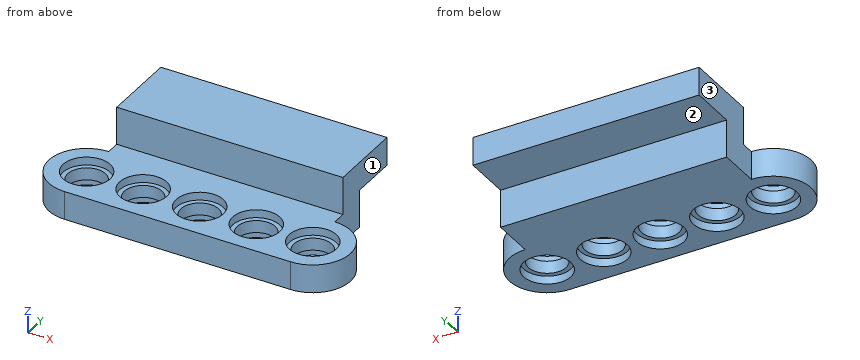
Autodesk Inventor part; units mm, degrees
ref_plane "YZ Plane" through (0, 0, 0) normal (1, 0, 0) x (0, 1, 0)
ref_plane "XZ Plane" through (0, 0, 0) normal (0, 1, 0) x (-1, 0, 0)
ref_plane "XY Plane" through (0, 0, 0) normal (0, 0, 1) x (1, 0, 0)
sketch "Sketch1" plane through (0, 0, 0) normal (0, 0, 1) x (1, 0, 0)
  arc A0 (-15, 4) -> (-15, -4) centre (-15, 0) ccw
  line L0 (-5, -4) -> (-15, -4)
  line L1 (-3, 0) -> (-3, 5.2247) construction
  arc A1 (9, -4) -> (9, 4) centre (9, 0) ccw
  line L2 (-5, -4) -> (9, -4)
  line L3 (9, 8.4612) -> (-15, 8.4612)
  line L4 (-15, 8.4612) -> (-15, 4)
  line L5 (9, 4) -> (9, 8.4612)
  dimension "d11" = 4
extrude "Extrusion1" add sketch "Sketch1" along normal blind 3
sketch "Sketch2" plane through (0, 0, 3) normal (0, 0, 1) x (1, 0, 0)
  arc A0 (-15, 4) -> (-15, -4) centre (-15, 0) ccw
  point P0 (0, 0)
hole "Hole1" at (-15, 0, 3) direction (0, 0, -1) diameter 4 depth 3 tip angle 118 counterbore diameter 5 counterbore depth 0.85
sketch "Sketch5" plane through (0, 0, 0) normal (0, 0, -1) x (-1, 0, 0)
  circle A0 centre (15, 0) radius 2
  circle A1 centre (15, 0) radius 2.5
  point P0 (0, 0)
extrude "Extrusion3" cut sketch "Sketch5" against normal blind 0.85
pattern_linear "Rectangular Pattern2" count 5 spacing 6 along (1, 0, 0) of "Extrusion3", "Hole1"
sketch "Sketch6" plane through (0, 0, 3) normal (0, 0, 1) x (1, 0, 0)
  point P0 (0, 0)
sketch "Sketch7" plane through (0, 0, 3) normal (0, 0, 1) x (1, 0, 0)
  line L0 (9, 4) -> (9, 8.4612)
  line L1 (-15, 8.4612) -> (9, 8.4612)
  line L2 (9, 8.4612) -> (9, 5.4612)
  line L3 (9, 5.4612) -> (-15, 5.4612)
  line L4 (-15, 5.4612) -> (-15, 8.4612)
  point P0 (0, 0)
  dimension "d24" = 3
extrude "Extrusion4" add sketch "Sketch7" along normal blind 4
sketch "Sketch8" plane through (-15, 8.4612, 0) normal (0, 1, 0) x (1, 0, 0)
  line L0 (24, -3) -> (24, -7)
  line L1 (0, -7) -> (24, -7)
  line L2 (24, -7) -> (24, -4)
  line L3 (24, -4) -> (0, -4)
  line L4 (0, -4) -> (0, -7)
  point P0 (15, 0)
  dimension "d27" = 3
extrude "Extrusion5" add sketch "Sketch8" along normal blind 5
properties part number "caster_pad"
Input: part model. Units: mm. Frame: model coordinates. Face numbers are marked on the shaded views. A direction names the side the tool comes from. Coordinates: 2 decimals unless noted, no trailing zeros. Loops run counter-clockwise (first coordinate to the right, second up) from the corner with the lowest first, then second, coordinate; pieces in that order, holes last. Notation, with made-up numbers: (47, -16) - (86, -16) arc R35 cw to (86, 22) - close; hole circle Ø8 at (69, -25.5). An arc over 180 degrees is marked (long way). Answer in a Markdown table with one row per item. Add a question column.
Item 1: Access query for the marked faces 1, 2 and 3. Directions: +Z, -Z, +X, -X, +Y, -Y. A direction counts if a zero-diameter tool reaches every point of the face in a straight line with its end or side. Return the directions, or none.
Item 2: Section query D-D on z = 5.75. Return the cut outline in (x, y), then the cut area to 3 significant figures.
Item 3: Contact query for flat-ended pins moving along their axis: P1, Ø1, axis at x = -14, y = -1.5, coming from the -Z side; P2, Ø2, axis at y = 6.5, z = 6, coming from the +X side; P3, Ø3, axis at y = 10, z = 5.5, coming from the -X side. Output: stop coordinate, or through.
Item 4: Section query B-B on y = 0. State how many separate pieces and enclosed holes the cut face has, then the cut area to 3 significant figures.
Item 5: Line query: line 1 along X through (y, z) = (0, 1.35); line 2 along X through (y, z) = (0, 2.6); line 3 along Y through (x, z) = (3, 0.25). Output: solid intervals per line, ascending. Write a range as [from, to].
Item 6: Section query C-C on y = 10. Return the cut outline in (x, z), then the cut area to 3 significant figures.
Item 7: Section query A-A on x = -6. Return the cut outline in (y, z).
Recorded:
| question | item | result |
|---|---|---|
| 1 | face 1 | +Z, -Z, +X, +Y |
| 1 | face 2 | -Z, +X, -X, +Y |
| 1 | face 3 | +Z, -Z, -X, +Y |
| 2 | outline | (-15, 5.46) - (9, 5.46) - (9, 13.46) - (-15, 13.46) - close |
| 2 | area | 192 mm^2 |
| 3 | P1 | z = 0.85 |
| 3 | P2 | x = 9 |
| 3 | P3 | x = -15 |
| 4 | separate pieces | 6 |
| 4 | enclosed holes | 0 |
| 4 | area | 27.5 mm^2 |
| 5 | line 1 | [-19, -17], [-13, -11], [-7, -5], [-1, 1], [5, 7], [11, 13] |
| 5 | line 2 | [-19, -17.5], [-12.5, -11.5], [-6.5, -5.5], [-0.5, 0.5], [5.5, 6.5], [11.5, 13] |
| 5 | line 3 | [-4, -2.5], [2.5, 8.46] |
| 6 | outline | (-15, 4) - (9, 4) - (9, 7) - (-15, 7) - close |
| 6 | area | 72.0 mm^2 |
| 7 | outline | (-4, 0) - (8.46, 0) - (8.46, 4) - (13.46, 4) - (13.46, 7) - (5.46, 7) - (5.46, 3) - (-4, 3) - close |
